```python
from build123d import *

# Parameters (mm, degrees)
SKETCH_1_R               = 41.5
SKETCH_1_R_2             = 33.15
EXTRUDE_1_DEPTH          = 8
SKETCH_2_R               = 1.55
CUT_EXTRUDE_1_DEPTH      = 8
PATTERN_CIRCULAR_1_COUNT = 12
SKETCH_3_R               = 33.15
SKETCH_3_R_2             = 29.5
EXTRUDE_2_DEPTH          = 2.5
CHAMFER_1_SIZE           = 2
SKETCH_4_R               = 1.55
CUT_EXTRUDE_8_DEPTH      = 4
PATTERN_CIRCULAR_7_COUNT = 12


with BuildPart() as part:
    # 草图1 → 凸台-拉伸1 (new body)
    with BuildSketch(Plane(origin=(0, 0, 0), x_dir=(0, 0, -1), z_dir=(1, 0, 0))):
        Circle(SKETCH_1_R)
        Circle(SKETCH_1_R_2, mode=Mode.SUBTRACT)
    extrude(amount=EXTRUDE_1_DEPTH)

    # 草图2 → 切除-拉伸1 (cut)
    with BuildSketch(Plane.ZY):
        with Locations((0, 37)):
            Circle(SKETCH_2_R)
    cut_extrude_1 = extrude(amount=-CUT_EXTRUDE_1_DEPTH, mode=Mode.SUBTRACT)

    # 阵列(圆周)1: 切除-拉伸1 ×12 about axis
    pattern_circular_1_axis = Axis((0, 0, 0), (1, 0, 0))
    for i in range(1, PATTERN_CIRCULAR_1_COUNT):
        add(cut_extrude_1.rotate(pattern_circular_1_axis, i * 360 / PATTERN_CIRCULAR_1_COUNT), mode=Mode.SUBTRACT)

    # 草图3 → 凸台-拉伸2 (add)
    with BuildSketch(Plane(origin=(8, 0, 0), x_dir=(0, 0, -1), z_dir=(1, 0, 0))):
        Circle(SKETCH_3_R)
        Circle(SKETCH_3_R_2, mode=Mode.SUBTRACT)
    extrude(amount=-EXTRUDE_2_DEPTH)

    # 倒角1
    chamfer_1_edges = [part.edges().sort_by_distance(p)[0] for p in [
        (8, 0, 41.5),
    ]]
    chamfer(chamfer_1_edges, length=CHAMFER_1_SIZE)

    # 草图4 → 切除-拉伸8 (cut)
    with BuildSketch(Plane(origin=(8, 0, 0), x_dir=(0, 0, -1), z_dir=(1, 0, 0))):
        with BuildLine():
            Line((39.393400463, 2.9), (37, 2.9))
            ThreePointArc((37, 2.9), (34.1, 0), (37, -2.9))
            Line((37, -2.9), (39.393400463, -2.9))
            ThreePointArc((39.393400463, -2.9), (39.473341119, -1.450979278), (39.5, 0))
            ThreePointArc((39.5, 0), (39.473341119, 1.450979278), (39.393400463, 2.9))
        make_face()
        with Locations((37, 0)):
            Circle(SKETCH_4_R, mode=Mode.SUBTRACT)
        with BuildLine():
            Line((45, 2.9), (39.393400463, 2.9))
            ThreePointArc((39.393400463, 2.9), (39.473341119, 1.450979278), (39.5, 0))
            ThreePointArc((39.5, 0), (39.473341119, -1.450979278), (39.393400463, -2.9))
            Line((39.393400463, -2.9), (45, -2.9))
            ThreePointArc((45, -2.9), (47.9, 0), (45, 2.9))
        make_face()
    cut_extrude_8 = extrude(amount=-CUT_EXTRUDE_8_DEPTH, mode=Mode.SUBTRACT)

    # 阵列(圆周)7: 切除-拉伸8 ×12 about axis
    pattern_circular_7_axis = Axis((0, 0, 0), (1, 0, 0))
    for i in range(1, PATTERN_CIRCULAR_7_COUNT):
        add(cut_extrude_8.rotate(pattern_circular_7_axis, i * 360 / PATTERN_CIRCULAR_7_COUNT), mode=Mode.SUBTRACT)


solid = part.part
```
CAD build for the part. Positions are in the model's coordinates, mm. A direction names the side the tool comes from. Round coordinates to 2 decimals unless told otherwise and drop trailing zeros. Loops run counter-clockwise (first coordinate to the right, second up) from the corner with the lowest first, then second, coordinate; pieces in that order, holes last. Notation, with made-up numbers: M -15,79 L -11,79 A11 cw -11,99 Z; hole C 69,73.25 d9. An arc over 180 degrees is marked long. Return JSON: item names as keys, results as strings. Group by question number.
(1) Drop flat-ended pins along their axis: P1, Ø1.5, axis at x = 1.5, z = 15, coming from the -Y side; P2, Ø1.5, axis at x = 1, y = -28.5, coming from the +Z side; P3, Ø3, axis at x = 6, z = -38, coming from the +Y side; P4, Ø2, axis at y = 32.5, z = 5.5, coming from the -X side. Give the stop position or say it passes through.
(2) Saw through at A-A, the plane y = 0. List the corners of the cut face in (x, z).
(3) Wall check: probe 1 along Y at (x, z) = (1.4, 0); probe 2 along Z at (x, y) = (6.75, -31); probe 3 along Y at (x, z) = (1.45, -37). Give the ranges that are in metal, low to high. Write a range as [from, to].
(4) Saw through at C-C, the plane x = 2. Give the number of separate pieces and of enclosed holes in the cut face, and give its area (3 significant figures).
(5) Mould opens along Y. For faces 6 (the flat face through (6, -39, 2.9)), 7 (the flat face through (6.028, -32.524, -22.127)), 8 (the cylindrical face through (6.03, 29.56, -17)) say: +Y half, -Y half, draft (parallel to the pull), parting line (faces both ways), or undercut.
(6) Tool access for faces 1 (the flat face through (4, 0, -39)), 2 (the cylindrical face through (2.71, -32.36, 7.19)), 3 (the flat face through (4, -19, -34)), 4 (the cylindrical face through (2, 17.2, 31.2)), 5 (the flat face through (6.028, -32.471, 22.096)): list every direction of +Z, -Z, +X, -X, +Y, -Y with a clear straight run to the whole face (end or side of a thin tool).
Answer list:
{
 "1": {"P1": "y = -38.98", "P2": "z = 30.86", "P3": "y = 18.19", "P4": "x = 0"},
 "2": {"outline": "M 0,-41.5 L 4,-41.5 L 4,-38.55 L 0,-38.55 Z; M 0,-35.45 L 4,-35.45 L 4,-34.1 L 8,-34.1 L 8,-29.5 L 5.5,-29.5 L 5.5,-33.15 L 0,-33.15 Z; M 0,33.15 L 5.5,33.15 L 5.5,29.5 L 8,29.5 L 8,34.1 L 4,34.1 L 4,35.45 L 0,35.45 Z; M 0,38.55 L 4,38.55 L 4,41.5 L 0,41.5 Z"},
 "3": {"probe 1": "[-41.5, -38.55], [-35.45, -33.15], [33.15, 35.45], [38.55, 41.5]", "probe 2": "[-26.45, -21.25], [-15.79, 15.79], [21.25, 26.45]", "probe 3": "[-18.79, -1.55], [1.55, 18.79]"},
 "4": {"separate pieces": "1", "enclosed holes": "13", "area": "1,870 mm2"},
 "5": {"face 6": "draft", "face 7": "-Y half", "face 8": "undercut"},
 "6": {"face 1": "-Z, +X", "face 2": "-X", "face 3": "+X", "face 4": "+X, -X", "face 5": "+X, -Y"}
}
